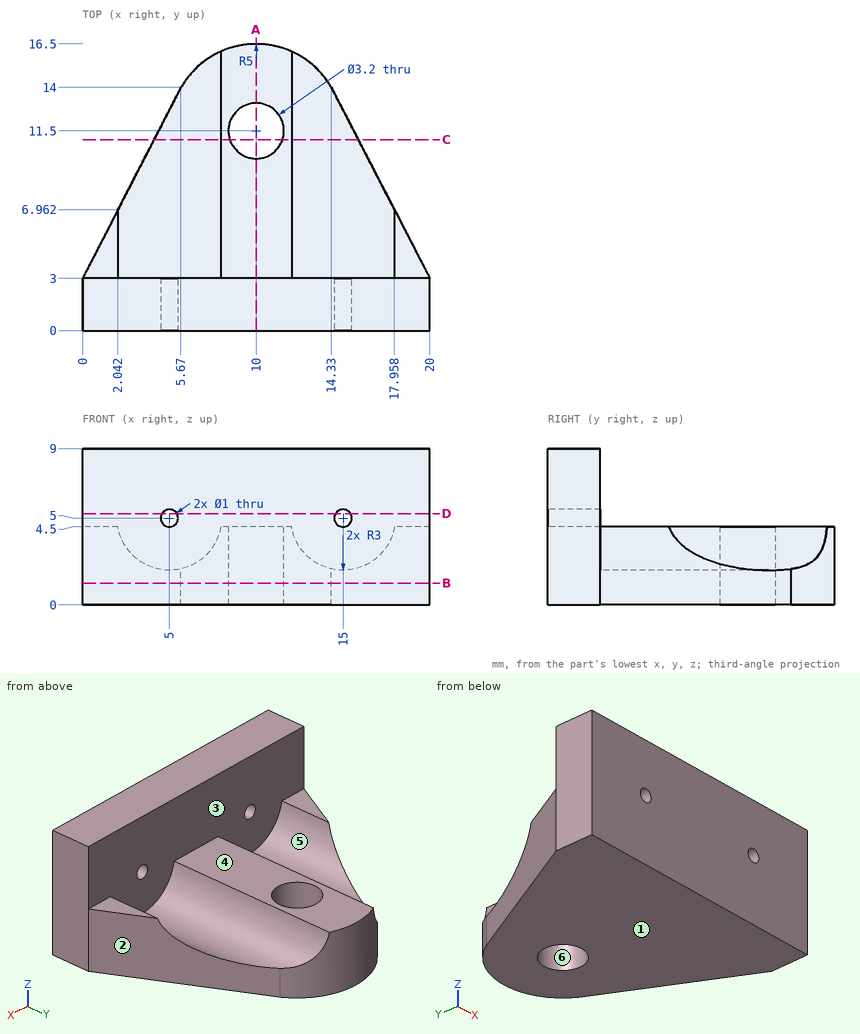
Study the drawing (mm; zero at the part's minimum x, y, z) and answer. A direction names the side the tool comes from. Give positions to 0.01 mm unless a question says otherwise; leave off trailing zeros. Order: outer loops, then holes, each group sorted by start corner. A loop starts at its lowest first (then second) coordinate and runs counter-clockwise, first axis right, second up.
1. Section C-C, the plane y = 11 is taken. Determine the outline of the cut face in (x, z).
Result sheet:
outline: (4.12, 0) - (8.48, 0) - (8.48, 4.5) - (7.96, 4.5) arc R3 cw to (4.12, 2.13) - close; (11.52, 0) - (15.88, 0) - (15.88, 2.13) arc R3 cw to (12.04, 4.5) - (11.52, 4.5) - close
2. Section B-B, the plane z = 1.25 is taken. Determine the outline of the cut face in (x, y), and give its area (3 significant figures).
Result sheet:
outline: (0, 0) - (20, 0) - (20, 3) - (14.33, 14) arc R5 ccw to (5.67, 14) - (0, 3) - close; hole circle Ø3.2 at (10, 11.5)
area: 225 mm2
3. Section A-A, the plane x = 10 is taken. Determine the outline of the cut face in (y, z).
Result sheet:
outline: (0, 0) - (9.9, 0) - (9.9, 4.5) - (3, 4.5) - (3, 9) - (0, 9) - close; (13.1, 0) - (16.5, 0) - (16.5, 4.5) - (13.1, 4.5) - close
4. For the marked faces 4, 5 and 6, determine the directions among +Z, -Z, +X, -X, +Y, -Y from which every point of the face is accessible in a straight line to the end or side of a thin tool.
Result sheet:
face 4: +Z, +X, -X, +Y
face 5: +Z, +Y
face 6: +Z, -Z
5. The mould has two halves that part along X. Classify the marked faces 1, 2 and 3: released by +X, released by -X, zero draft, split by the parting line, or undercut.
Result sheet:
face 1: zero draft
face 2: released by +X
face 3: undercut
6. Each of these flat-tipped pins is pushed along its axis until it touches: P1, Ø2, axis at x = 12, y = 13.5, coming from the +Z side; P2, Ø5, axis at x = 11.5, z = 7.5, coming from the +Y side. Where does it stop, or does it pass through?
Result sheet:
P1: stops at z = 4.5
P2: stops at y = 3
7. Straight lines are drawn through the part: L1, parallel to Y at x = 10, z = 3.4; L2, parallel to Z at x = 5, y = 2; L3, parallel to Y at x = 12.5, z = 4.5. For each, find the intervals that lie inside material, in ascending order.
Result sheet:
L1: y = 0 to 9.9, 13.1 to 16.5
L2: z = 0 to 4.5, 5.5 to 9
L3: y = 0 to 3
8. Section D-D, the plane z = 5.25 is taken. Determine the outline of the cut face in (x, y).
Result sheet:
outline: (0, 0) - (4.57, 0) - (4.57, 3) - (0, 3) - close; (5.43, 0) - (14.57, 0) - (14.57, 3) - (5.43, 3) - close; (15.43, 0) - (20, 0) - (20, 3) - (15.43, 3) - close
